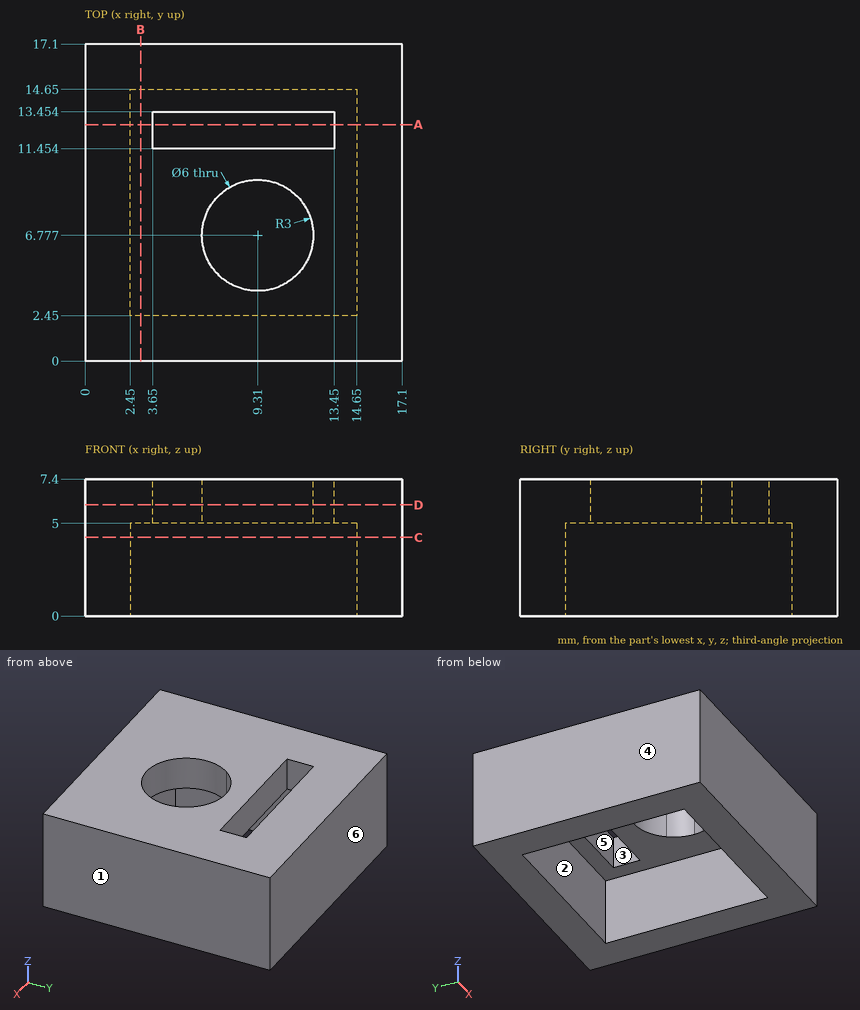
The figure shows three views and two pictorial views of one solid part (mm, origin at its lowest corner). Answer the questions. A direction names the side the tool comes from. Give positions to 0.01 mm unless a question says otherwise; leave off trailing zeros. Loops run counter-clockwise (first coordinate to the right, second up) from the corner with the lowest first, then second, coordinate; pieces in that order, holes last. Notation, with made-up numbers: M 4.5,5.25 L 35.5,5.25 A24 ccw 35.5,17.25 Z; hole C -36,61.25 d2. An arc over 180 degrees is marked long. Write each question's results on one line, items separated by ' | '.
1. Section C-C on z = 4.25 is taken. Give the vertices of the cut face in (x, y).
Values:
outline: M 0,0 L 17.1,0 L 17.1,17.1 L 0,17.1 Z; hole M 2.45,2.45 L 14.65,2.45 L 14.65,14.65 L 2.45,14.65 Z
2. Given pin 1 (6 mm diameter, centred on x = 8, y = 7, fed in from -Z); pin 2 (9.5 mm diameter, centred on x = 9.31, y = 6.78, fed in from +Z), each flat-ended and moving along its own axis, determine where each tip first touches the part or whether it passes through.
Values:
pin 1: stops at z = 5 | pin 2: stops at z = 7.4
3. Straight lines are drawn through the part: line 1 (Y direction, x = 12.5, z = 2.5); line 2 (X direction, y = 11.5, z = 6); line 3 (Y direction, x = 13, z = 7.25) (1 decimal). For each, find the intervals that lie inside material, in ascending order. Write a range as [from, to].
Values:
line 1: y = [0, 2.45], [14.65, 17.1] | line 2: x = [0, 3.65], [13.45, 17.1] | line 3: y = [0, 11.5], [13.5, 17.1]
4. Section A-A on y = 12.75 is taken. Give the vertices of the cut face in (x, z).
Values:
outline: M 0,0 L 2.45,0 L 2.45,5 L 3.65,5 L 3.65,7.4 L 0,7.4 Z; M 13.45,5 L 14.65,5 L 14.65,0 L 17.1,0 L 17.1,7.4 L 13.45,7.4 Z
5. Section B-B on x = 3 is taken. Give the vertices of the cut face in (y, z).
Values:
outline: M 0,0 L 2.45,0 L 2.45,5 L 14.65,5 L 14.65,0 L 17.1,0 L 17.1,7.4 L 0,7.4 Z
6. The mould has two halves that part along Y. Classify the marked faces 4, 5 and 6: pulls with the +Y half, pulls with the -Y half, needs draft (parallel to the pull), parting line crosses it, or undercut.
Values:
face 4: needs draft | face 5: undercut | face 6: pulls with the +Y half
7. Section D-D on z = 6 is taken. State how many separate pieces and enclosed holes the cut face has.
Values:
separate pieces: 1 | enclosed holes: 2
8. A tool of negligible diameter and unlimited length cuts with its end or side. For the marked faces 1, 2 and 3, from which of +Z, -Z, +X, -X, +Y, -Y can it reach the whole face along a straight path? Write none if from no direction.
Values:
face 1: +Z, -Z, +X, +Y, -Y | face 2: -Z | face 3: +Z, -Z
